```python
from build123d import *

# Parameters (mm, degrees)
BOSS_EXTRUDE1_DEPTH = 30
SKETCH3_R           = 22.5
BOSS_EXTRUDE2_DEPTH = 10
FILLET2_R           = 5
SKETCH4_R           = 3.5
CUT_EXTRUDE1_DEPTH  = 70


with BuildPart() as part:
    # Sketch1 → Boss-Extrude1 (new body)
    with BuildSketch(Plane(origin=(0, 0, 0), x_dir=(0, 0, -1), z_dir=(1, 0, 0))):
        Polygon((0, 0), (0, -65), (54, -65), (54, 0), (49.5, 0), (49.5, -55), (4.5, -55), (4.5, 0), align=None)
    extrude(amount=BOSS_EXTRUDE1_DEPTH)

    # Sketch3 → Boss-Extrude2 (add)
    with BuildSketch(Plane.XZ.offset(65)):
        with Locations((15, -27)):
            Circle(SKETCH3_R)
    extrude(amount=-BOSS_EXTRUDE2_DEPTH)

    # Fillet2
    fillet2_edges = [part.edges().sort_by_distance(p)[0] for p in [
        (0, 0, -2.25),
        (15, -55, -4.5),
        (15, -55, -49.5),
        (15, -65, -54),
        (15, -65, 0),
        (30, 0, -51.75),
        (30, 0, -2.25),
        (0, 0, -51.75),
    ]]
    fillet(fillet2_edges, radius=FILLET2_R)

    # Sketch4 → Cut-Extrude1 (cut)
    with BuildSketch(Plane(origin=(0, 0, -54), x_dir=(-1, 0, 0), z_dir=(0, 0, -1))):
        with Locations((-15, -26)):
            Circle(SKETCH4_R)
    extrude(amount=-CUT_EXTRUDE1_DEPTH, mode=Mode.SUBTRACT)


solid = part.part
```
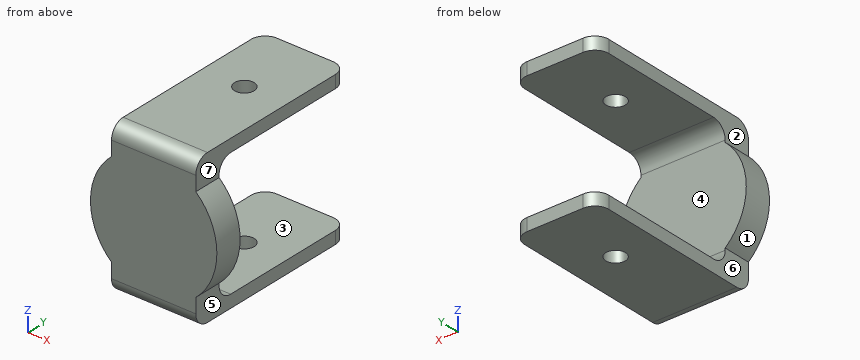
Input: part model. Units: mm. Frame: model coordinates. Face numbers are marked on the shaded views. A direction names the side the tool comes from. Give positions to 0.01 mm unless a question says otherwise; leave off trailing zeros. Order: outer loops, then holes, each group sorted by start corner. A loop starts at its lowest first (then second) coordinate and runs counter-clockwise, first axis right, second up.
1. Section A-A on y = -40.5. Return the cut outline in (x, z).
Derived:
outline: (0, -54) - (30, -54) - (30, -49.5) - (0, -49.5) - close; (0, -4.5) - (30, -4.5) - (30, 0) - (0, 0) - close
2. Section C-C on y = -26. Return the cut outline in (x, z).
Derived:
outline: (0, -54) - (11.5, -54) - (11.5, -49.5) - (0, -49.5) - close; (0, -4.5) - (11.5, -4.5) - (11.5, 0) - (0, 0) - close; (18.5, -54) - (30, -54) - (30, -49.5) - (18.5, -49.5) - close; (18.5, -4.5) - (30, -4.5) - (30, 0) - (18.5, 0) - close
3. Material intervals for L1, parallel to Z at x = 13, y = -47; L2, parallel to Y at x = 13.5, z = -11; L3, parallel to Z at x = 22, y = -53.5, sorted ascending.
Derived:
L1: z = -54 to -49.5, -4.5 to 0
L2: y = -65 to -55
L3: z = -54 to -48.07, -5.93 to 0
4. Reachability of the marked faces 4, 5, 6 and 7 from +Z, -Z, +X, -X, +Y, -Y: full face, straight path, thin tool, end or side. Return the list, or none.
Derived:
face 4: +X, -X, +Y
face 5: -Z, +X, +Y, -Y
face 6: -Z, -X, +Y, -Y
face 7: +Z, +X, +Y, -Y
5. Pin query (flat end, axial travel): pin 1 (9 mm diameter, centred on x = 15, y = -26, fed in from +Z); pin 2 (10.5 mm diameter, centred on x = 17, z = -26.5, fed in from +Y); pin 3 (11.5 mm diameter, centred on y = -39.5, z = -50, fed in from -X); pin 4 (5 mm diameter, centred on y = -43, z = -50.5, fed in from +X). Return the tip coordinate at first contact, or that it passes through.
Derived:
pin 1: stops at z = 0
pin 2: stops at y = -55
pin 3: stops at x = 0
pin 4: stops at x = 30
6. Section D-D on x = 2. Return the cut outline in (y, z), and give its area (3 significant figures).
Derived:
outline: (-65, -49) arc R5 ccw to (-60, -54) - (-1, -54) - (-1, -49.5) - (-50, -49.5) arc R5 cw to (-55, -44.5) - (-55, -9.5) arc R5 cw to (-50, -4.5) - (-1, -4.5) - (-1, 0) - (-60, 0) arc R5 ccw to (-65, -5) - close
area: 1,030 mm2
7. Section B-B on x = 15. Return the cut outline in (y, z).
Derived:
outline: (-65, -49) arc R5 ccw to (-60, -54) - (-29.5, -54) - (-29.5, -49.5) - (-50, -49.5) arc R5 cw to (-55, -44.5) - (-55, -9.5) arc R5 cw to (-50, -4.5) - (-29.5, -4.5) - (-29.5, 0) - (-60, 0) arc R5 ccw to (-65, -5) - close; (-22.5, -54) - (0, -54) - (0, -49.5) - (-22.5, -49.5) - close; (-22.5, -4.5) - (0, -4.5) - (0, 0) - (-22.5, 0) - close
8. Mould query, pull axis Z, two halves, no side actions, for the marked faces 1, 2 and 3. Classes: released by +Z, released by -Z, zero draft, split by the parting line, or undercut.
Derived:
face 1: split by the parting line
face 2: zero draft
face 3: undercut
